Geometry check sheet. Reference: the model listing, model coordinates, mm. Coordinates: 2 decimals unless noted, no trailing zeros. Write each loop counter-clockwise with the first axis right and the second up, starting at its lowest first coordinate (ties: lowest second). Pieces come first, ordered by that corner, then holes. Notation, with made-up numbers: (30, 9.5) -> (73, 9.5) arc R23 ccw to (73, 32.5) -> close; hole circle Ø10 at (78, 41). An arc over 180 degrees is marked (long way). One line per question, with ' | ' between items.
from build123d import *

# Parameters (mm, degrees)
SKETCH1_R          = 3.5
SKETCH1_W          = 81.6
SKETCH1_H          = 3
BASE_SHAPE_DEPTH   = 3
SKETCH2_R          = 2.65
MAGNET_HOLES_DEPTH = 1.1
MILLING_FILLETS_R  = 1


with BuildPart() as part:
    # Sketch1 → Base shape (new body)
    with BuildSketch(Plane(origin=(0, 0, 0), x_dir=(1, 0, 0), z_dir=(0, 1, 0))):
        with Locations((-35, 0)):
            Circle(SKETCH1_R)
        with Locations((35, 0)):
            Circle(SKETCH1_R)
        Rectangle(SKETCH1_W, SKETCH1_H)
    extrude(amount=BASE_SHAPE_DEPTH)

    # Sketch2 → Magnet holes (cut)
    with BuildSketch(Plane(origin=(0, 3, 0), x_dir=(1, 0, 0), z_dir=(0, 1, 0))):
        with Locations((-35, 0)):
            Circle(SKETCH2_R)
        with Locations((35, 0)):
            Circle(SKETCH2_R)
    extrude(amount=-MAGNET_HOLES_DEPTH, mode=Mode.SUBTRACT)

    # Milling fillets
    milling_fillets_edges = [part.edges().sort_by_distance(p)[0] for p in [
        (-38.16227766, 1.5, -1.5),
        (31.83772234, 1.5, -1.5),
        (38.16227766, 1.5, -1.5),
        (31.83772234, 1.5, 1.5),
        (38.16227766, 1.5, 1.5),
        (-31.83772234, 1.5, 1.5),
        (-38.16227766, 1.5, 1.5),
        (-31.83772234, 1.5, -1.5),
    ]]
    fillet(milling_fillets_edges, radius=MILLING_FILLETS_R)


solid = part.part
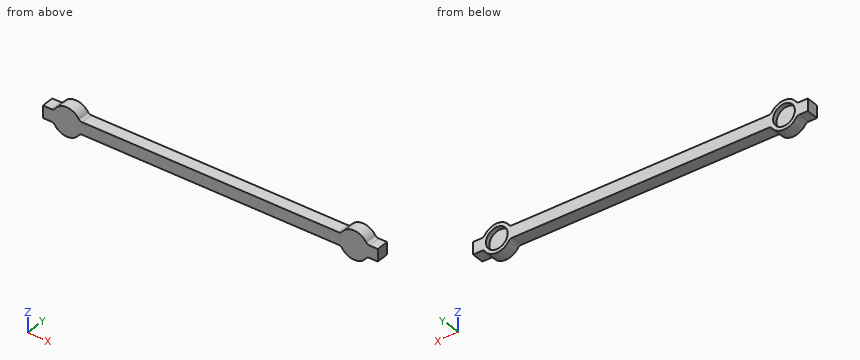
1. Cross-section at D-D on x = 1. Record the boundary of the cut face in (y, z).
Worked answers:
outline: (0, -1.5) -> (3, -1.5) -> (3, 1.5) -> (0, 1.5) -> close
2. Cross-section at B-B on x = -35. Record the boundary of the cut face in (y, z).
Worked answers:
outline: (0, -3.5) -> (3, -3.5) -> (3, -2.65) -> (1.9, -2.65) -> (1.9, 2.65) -> (3, 2.65) -> (3, 3.5) -> (0, 3.5) -> close
3. Material ranges on line 1 (X direction, y = 2.35, z = 0); line 2 (Z direction, x = 35, y = 2.1); line 3 (X direction, y = 2.5, z = 1.25), recorded low to high. Write a range as from..to.
Worked answers:
line 1: -40.8..-37.65, -32.35..32.35, 37.65..40.8 | line 2: -3.5..-2.65, 2.65..3.5 | line 3: -40.8..-37.34, -32.66..32.66, 37.34..40.8
4. Go/stop test with flat-tipped pins: P1, Ø2.5, axis at x = -34.5, z = -0.5, coming from the +Y side; P2, Ø1, axis at x = 39.5, y = 2, coming from the -Z side. Record where each tip stops, or that it passes through.
Worked answers:
P1: y = 1.9 | P2: z = -1.5
5. Cross-section at A-A on z = 0. Record the boundary of the cut face in (x, y), and give its area (3 significant figures).
Worked answers:
outline: (-40.8, 0) -> (40.8, 0) -> (40.8, 3) -> (37.65, 3) -> (37.65, 1.9) -> (32.35, 1.9) -> (32.35, 3) -> (-32.35, 3) -> (-32.35, 1.9) -> (-37.65, 1.9) -> (-37.65, 3) -> (-40.8, 3) -> close | area: 233 mm²
6. Cross-section at C-C on y = 1.45. Record the boundary of the cut face in (x, z).
Worked answers:
outline: (-40.8, -1.5) -> (-38.74, -1.5) arc R1 cw to (-37.91, -1.94) arc R3.5 ccw to (-32.09, -1.94) arc R1 cw to (-31.26, -1.5) -> (31.26, -1.5) arc R1 cw to (32.09, -1.94) arc R3.5 ccw to (37.91, -1.94) arc R1 cw to (38.74, -1.5) -> (40.8, -1.5) -> (40.8, 1.5) -> (38.74, 1.5) arc R1 cw to (37.91, 1.94) arc R3.5 ccw to (32.09, 1.94) arc R1 cw to (31.26, 1.5) -> (-31.26, 1.5) arc R1 cw to (-32.09, 1.94) arc R3.5 ccw to (-37.91, 1.94) arc R1 cw to (-38.74, 1.5) -> (-40.8, 1.5) -> close
